The listing builds one solid part. Answer for the finished solid, in the listing's coordinates (mm). Face numbers are marked on the shaded views. A direction names the side the tool comes from. Give positions to 0.01 mm unless a question says otherwise; leave off trailing zeros. Loops run counter-clockwise (first coordinate to the right, second up) from the corner with the lowest first, then second, coordinate; pieces in that order, holes last.
Item 1: Section D-D, the plane z = 51 is taken. Give the vertices of the cut face in (x, y), and give its area (3 significant figures).
Item 2: Section B-B, the plane z = 11 is taken. Give the number of separate pieces and of enclosed holes in the cut face, and give its area (3 significant figures).
Item 3: Each of these flat-tipped pins is pushed along its axis until it touches: pin 1 Ø10 at (x, y) = (84, -11) entering from +Z; pin 2 Ø1.5 at (x, y) = (124.5, -23.5) entering from -Z; pin 3 Ø8 at (y, z) = (-47.5, 42) entering from +X. Where does it stop, or does it pass through?
Item 4: Consider line 1 along Y through (x, z) = (69, 15); line 2 along Z through (x, y) = (100, -30); line 3 along X through (y, z) = (-29.5, 60). Determine where each line is inside the solid, lowest interval first.
Item 5: The mould has two halves that part along Y. Classify the marked faces 1, 2 and 3: pulls with the +Y half, pulls with the -Y half, needs draft (parallel to the pull), parting line crosses it, or undercut.
Item 6: Section C-C, the plane x = 172 is taken. Give the vertices of the cut face in (y, z), and give its area (3 significant figures).
Item 7: Section A-A, the plane x = 69.85 is taken. Give the vertices of the cut face in (y, z).
Item 8: A tool of negligible diameter and unlimited length cuts with its end or side. For the marked faces 4 and 5, from which of +Z, -Z, +X, -X, +Y, -Y can it reach the whole face along a straight path? Write none if from no direction.
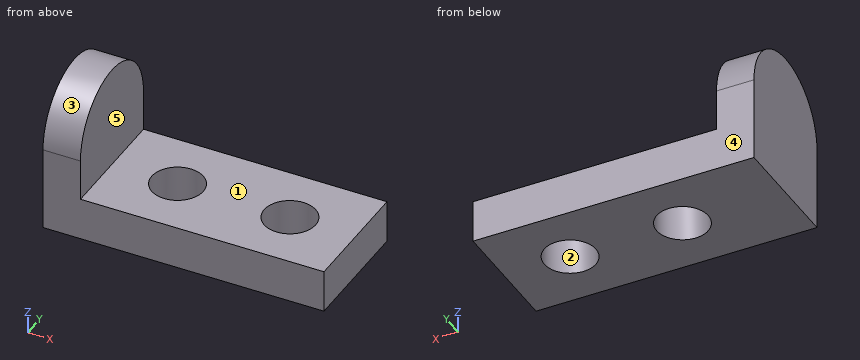
from build123d import *

# Parameters (mm, degrees)
F1_DEPTH = 82.55
F3_DEPTH = 190.501
F4_R     = 17.4625
F5_DEPTH = 29.01032


with BuildPart() as f1:
    # F0 (on Front) → F1 (new body)
    with BuildSketch(Plane.XZ):
        Polygon((0, 101.6), (0, 0), (190.5, 0), (190.5, 29.00932), (25.4, 29.00932), (25.4, 101.6), align=None)
    extrude(amount=F1_DEPTH)

    # F2 (on face) → F3 (cut, through all)
    with BuildSketch(Plane(origin=(0, 0, 0), x_dir=(0, -1, 0), z_dir=(-1, 0, 0))):
        with BuildLine():
            Line((0, 101.6), (0, 57.15))
            ThreePointArc((0, 57.15), (41.275, 98.425), (82.55, 57.15))
            Line((82.55, 57.15), (82.55, 101.6))
            Line((82.55, 101.6), (0, 101.6))
        make_face()
    extrude(amount=-F3_DEPTH, mode=Mode.SUBTRACT)

    # F4 (on face) → F5 (cut, through all)
    with BuildSketch(Plane.XY.offset(29.00932)):
        with Locations((69.85, -41.275)):
            Circle(F4_R)
        with Locations((146.05, -41.275)):
            Circle(F4_R)
    extrude(amount=-F5_DEPTH, mode=Mode.SUBTRACT)


solid = f1.part
Worked answers:
1. outline: (0, -82.55) - (25.4, -82.55) - (25.4, 0) - (0, 0) - close
1. area: 2,100 mm2
2. separate pieces: 1
2. enclosed holes: 2
2. area: 13,800 mm2
3. pin 1: stops at z = 29.01
3. pin 2: stops at z = 0
3. pin 3: stops at x = 25.4
4. line 1: y = -82.55 to -58.72, -23.83 to 0
4. line 2: z = 0 to 29.01
4. line 3: x = 0 to 25.4
5. face 1: needs draft
5. face 2: undercut
5. face 3: parting line crosses it
6. outline: (-82.55, 0) - (0, 0) - (0, 29.01) - (-82.55, 29.01) - close
6. area: 2,390 mm2
7. outline: (-82.55, 0) - (-58.74, 0) - (-58.74, 29.01) - (-82.55, 29.01) - close; (-23.81, 0) - (0, 0) - (0, 29.01) - (-23.81, 29.01) - close
8. face 4: +Z, -Z, +X, -X, +Y
8. face 5: +Z, +X, +Y, -Y
